```python
from build123d import *

# Parameters (mm, degrees)
F0_W     = 25.4
F0_H     = 12.7
F1_DEPTH = 2.54
F2_W     = 1.27
F2_H     = 8.89
F3_DEPTH = 2.54
F4_W     = 8.89
F4_H     = 1.27
F5_DEPTH = 1.27


with BuildPart() as f1:
    # F0 (on Top) → F1 (new body)
    with BuildSketch(Plane.XY):
        Rectangle(F0_W, F0_H)
    extrude(amount=F1_DEPTH)

    # F2 (on face) → F3 (join)
    with BuildSketch(Plane.XY.offset(2.54)):
        with Locations((-11.43, 0)):
            Rectangle(F2_W, F2_H)
    extrude(amount=F3_DEPTH)

    # F4 (on face) → F5 (join)
    with BuildSketch(Plane(origin=(-12.065, 0, 0), x_dir=(0, -1, 0), z_dir=(-1, 0, 0))):
        with Locations((0, 4.445)):
            Rectangle(F4_W, F4_H)
    extrude(amount=F5_DEPTH)


solid = f1.part
```
Source: CAD feature listing. Evaluate the final solid. Frame: model axes, mm. A direction names the side the tool comes from. Round coordinates to 2 decimals unless told otherwise and drop trailing zeros. Loops run counter-clockwise (first coordinate to the right, second up) from the corner with the lowest first, then second, coordinate; pieces in that order, holes last. Notation, with made-up numbers: M 56,65 L 109,65 A10 cw 109,78 Z; hole C 16.25,-21 d11. An arc over 180 degrees is marked long. Use a Markdown table: item, result. Add a question column.
1. Set-up query: faces 1 (the flat face through (-12.7, 0, 1)), 2 (the flat face through (-12, -4.445, 4)), 3 (the flat face through (-10.795, 0, 4)), 4 (the flat face through (-12, 4.445, 4)), 5 (the flat face through (-13, 0, 3.81)). Return all of +Z, -Z, +X, -X, +Y, -Y with unobstructed straight access to the full face (end or side cutting, diameter ignored); none if empty.
2. Contact query for flat-ended pins moving along their axis: pin 1 (1.5 mm diameter, centred on x = -9.5, y = 0, fed in from +Z); pin 2 (1 mm diameter, centred on x = 10, z = 4, fed in from -Y); pin 3 (2 mm diameter, centred on y = -2, z = 1.5, fed in from -X); pin 4 (2 mm diameter, centred on x = -11.5, z = 4, fed in from -Y) (3 decimals). Output: stop coordinate, or through.
3. Cut plane B-B, the plane z = 0.45. Output: boundary loops of the cut face in (x, y), and give its area (3 significant figures).
4. Cut plane A-A, the plane y = 0.5. Output: boundary loops of the cut face in (x, z) (3 decimals), and give its area (3 significant figures).
5. Cut plane C-C, the plane x = 7.25. Output: boundary loops of the cut face in (y, z).
6. Ray query, line 1 along Z through (x, y) = (-2.25, -1.25); line 2 along X through (y, z) = (1, 1.5); line 3 along X through (y, z) = (1, 4.7) (3 decimals). Return the intervals inside material, ascending. Write a range as [from, to].
Solution:
| question | item | result |
|---|---|---|
| 1 | face 1 | -Z, -X, +Y, -Y |
| 1 | face 2 | +Z, +X, -X, -Y |
| 1 | face 3 | +Z, +X, +Y, -Y |
| 1 | face 4 | +Z, +X, -X, +Y |
| 1 | face 5 | -X, +Y, -Y |
| 2 | pin 1 | stops at z = 2.54 |
| 2 | pin 2 | passes through |
| 2 | pin 3 | stops at x = -12.7 |
| 2 | pin 4 | stops at y = -4.445 |
| 3 | outline | M -12.7,-6.35 L 12.7,-6.35 L 12.7,6.35 L -12.7,6.35 Z |
| 3 | area | 323 mm2 |
| 4 | outline | M -13.335,3.81 L -12.065,3.81 L -12.065,2.54 L -12.7,2.54 L -12.7,0 L 12.7,0 L 12.7,2.54 L -10.795,2.54 L -10.795,5.08 L -13.335,5.08 Z |
| 4 | area | 69.4 mm2 |
| 5 | outline | M -6.35,0 L 6.35,0 L 6.35,2.54 L -6.35,2.54 Z |
| 6 | line 1 | z = [0, 2.54] |
| 6 | line 2 | x = [-12.7, 12.7] |
| 6 | line 3 | x = [-13.335, -10.795] |
